For this review, take the finished solid that the model builds, in its own axes (mm). Coordinates: 2 decimals unless noted, no trailing zeros. Order: outer loops, then holes, each group sorted by start corner. A loop starts at its lowest first (then second) coordinate and runs counter-clockwise, first axis right, second up.
Autodesk Inventor part; units mm, degrees
ref_plane "YZ Plane" through (0, 0, 0) normal (1, 0, 0) x (0, 1, 0)
ref_plane "XZ Plane" through (0, 0, 0) normal (0, 1, 0) x (-1, 0, 0)
ref_plane "XY Plane" through (0, 0, 0) normal (0, 0, 1) x (1, 0, 0)
sketch "Sketch1" plane through (0, 0, 0) normal (1, 0, 0) x (0, 1, 0)
  line L0 (0, 0) -> (20, 0)
  line L1 (20, 0) -> (20, 40) construction
  line L2 (20, 40) -> (0, 40)
  line L3 (0, 40) -> (0, 0)
  line L4 (20, 0) -> (65, 0) construction
  line L5 (48.2843, 28.2843) -> (36.5685, 40)
  line L6 (36.5685, 40) -> (20, 40)
  line L7 (48.2843, 28.2843) -> (20, 0) construction
  line L8 (20, 0) -> (48.2843, -28.2843)
  line L9 (48.2843, -28.2843) -> (76.5685, 0)
  line L10 (76.5685, 0) -> (48.2843, 28.2843)
  line L11 (10, 40) -> (10, 0) construction
  circle A0 centre (10, 30) radius 2.6
  circle A1 centre (10, 10) radius 2.6
  line L12 (48.2843, 14.1421) -> (34.1421, 0) construction
  line L13 (34.1421, 0) -> (48.2843, -14.1421) construction
  line L14 (48.2843, -14.1421) -> (62.4264, 0) construction
  line L15 (62.4264, 0) -> (48.2843, 14.1421) construction
  circle A2 centre (62.4264, 0) radius 2.6
  circle A3 centre (48.2843, 14.1421) radius 2.6
  circle A4 centre (34.1421, 0) radius 2.6
  circle A5 centre (48.2843, -14.1421) radius 2.6
  dimension "d0" = 20
  dimension "d1" = 40
  dimension "d2" = 40
  dimension "d4" = 40
  dimension "d5" = 45
  dimension "d6" = 5.2
  dimension "d7" = 5.2
  dimension "d8" = 10
  dimension "d9" = 10
  dimension "d10" = 20
  dimension "d11" = 20
  dimension "d12" = 10
  dimension "d13" = 10
  dimension "d14" = 5.2
  dimension "d15" = 5.2
  dimension "d16" = 5.2
  dimension "d17" = 5.2
extrude "Extrusion1" add sketch "Sketch1" along normal blind 3.175
chamfer "Chamfer1" distance 10 angle 45 1 edges at (1.5875, 20, 0)
chamfer "Chamfer2" distance 3 angle 45 4 edges at (1.5875, 48.2843, -28.2843) (1.5875, 76.5685, 0) (1.5875, 0, 0) (1.5875, 0, 40)
equation "\"d7\" = d6"
equation "\"d14\" = d6"
equation "\"d15\" = d6"
equation "\"d16\" = d6"
equation "\"d17\" = d6"
properties part number "45deg 2040 Connector Bracket"
1. Clearance check with flat-ended pins moving along their axes: pin 1 Ø4.5 at (y, z) = (10, 30) entering from +X; pin 2 Ø1 at (x, y) = (2.5, 51) entering from -Z; pin 3 Ø1 at (x, y) = (1.5, 8) entering from -Z. State where each tip first meets the part, or that it passes through.
Answer below:
pin 1: passes through
pin 2: stops at z = -26.07
pin 3: stops at z = 0
2. Take a section at D-D, the plane z = -20. Give the boundary of the cut face in (x, y) (3 decimals), plus the area to 3 significant figures.
Answer below:
outline: (0, 40) - (3.175, 40) - (3.175, 56.569) - (0, 56.569) - close
area: 52.6 mm2
3. Take a section at B-B, the plane y = 61. Give the boundary of the cut face in (x, z) (3 decimals), plus the area to 3 significant figures.
Answer below:
outline: (0, -15.569) - (3.175, -15.569) - (3.175, -2.174) - (0, -2.174) - close; (0, 2.174) - (3.175, 2.174) - (3.175, 15.569) - (0, 15.569) - close
area: 85.1 mm2
4. The part is to be moulded in two halves that separate along Y. For faces 1 (the face through (2, 36, -16)), 2 (the face through (1.565, 50.764, -14.923)), 3 (the face through (2, 6, 0)), say which applies: +Y half, -Y half, draft (parallel to the pull), parting line (faces both ways), or undercut.
Answer below:
face 1: -Y half
face 2: undercut
face 3: draft
5. Take a section at C-C, the plane y = 69. Give the boundary of the cut face in (x, z) (3 decimals).
Answer below:
outline: (0, -7.569) - (3.175, -7.569) - (3.175, 7.569) - (0, 7.569) - close
6. To check wall thickness, follow L1, parallel to Z at x = 1.9, y = 47.5; L2, parallel to Y at x = 0.8, z = -1; L3, parallel to Y at x = 3.05, z = 2. State the ranges of each line that lie inside material, in increasing order.
Answer below:
L1: z = -26.16 to -16.62, -11.66 to 11.66, 16.62 to 29.07
L2: y = 12.41 to 31.74, 36.54 to 60.03, 64.83 to 74.45
L3: y = 1 to 32.48, 35.8 to 60.77, 64.09 to 74.45
7. Take a section at A-A, the plane z = 30. Give the boundary of the cut face in (x, y) (3 decimals).
Answer below:
outline: (0, 0) - (3.175, 0) - (3.175, 7.4) - (0, 7.4) - close; (0, 12.6) - (3.175, 12.6) - (3.175, 46.569) - (0, 46.569) - close
